The figure shows three views and two pictorial views of one solid part (mm, origin at its lowest corner). Answer the questions. Give positions to 0.01 mm unless a question says otherwise; leave off trailing zeros. Loops run counter-clockwise (first coordinate to the right, second up) from the corner with the lowest first, then second, coordinate; pieces in that order, holes last. Notation, with made-up numbers: (-9.5, 62) - (31.5, 62) arc R23 cw to (31.5, 83) - close; hole circle Ø5 at (76, 81). An arc over 180 degrees is marked (long way). Use a Markdown table: item, result. Add a question column.
Item 1: For a pull along X with two mould halves and no side action, classify the marked faces 1, 2, 3 and 4 as +X half, -X half, draft (parallel to the pull), parting line (faces both ways), or undercut.
Item 2: Consider probe 1 along X at (y, z) = (2, 19); probe 2 along X at (y, z) = (12, 19.5); probe 3 along X at (y, z) = (48, 18). Determine where each line is inside the solid, lowest interval first. Write a range as [from, to].
Item 3: A cutting plane is placed at A-A (z = 19.05). Determine the outline of the cut face in (x, y) (3 decimals), plus the area to 3 significant figures.
Item 4: A cutting plane is placed at B-B (x = 120.65). Determine the outline of the cut face in (y, z) (3 decimals).
Item 5: Each of these flat-tipped pins is pushed along its axis until it touches: P1, Ø17, axis at x = 120.65, z = 19.05, coming from the -Y side; P2, Ø3, axis at x = 78, z = 17, coming from the -Y side. Where does it stop, or does it pass through?
Item 6: A cutting plane is placed at D-D (y = 21.5). Determine the outline of the cut face in (x, z) (3 decimals), plus the area to 3 significant figures.
Item 7: A cutting plane is placed at C-C (x = 59.69). Determine the outline of the cut face in (y, z).
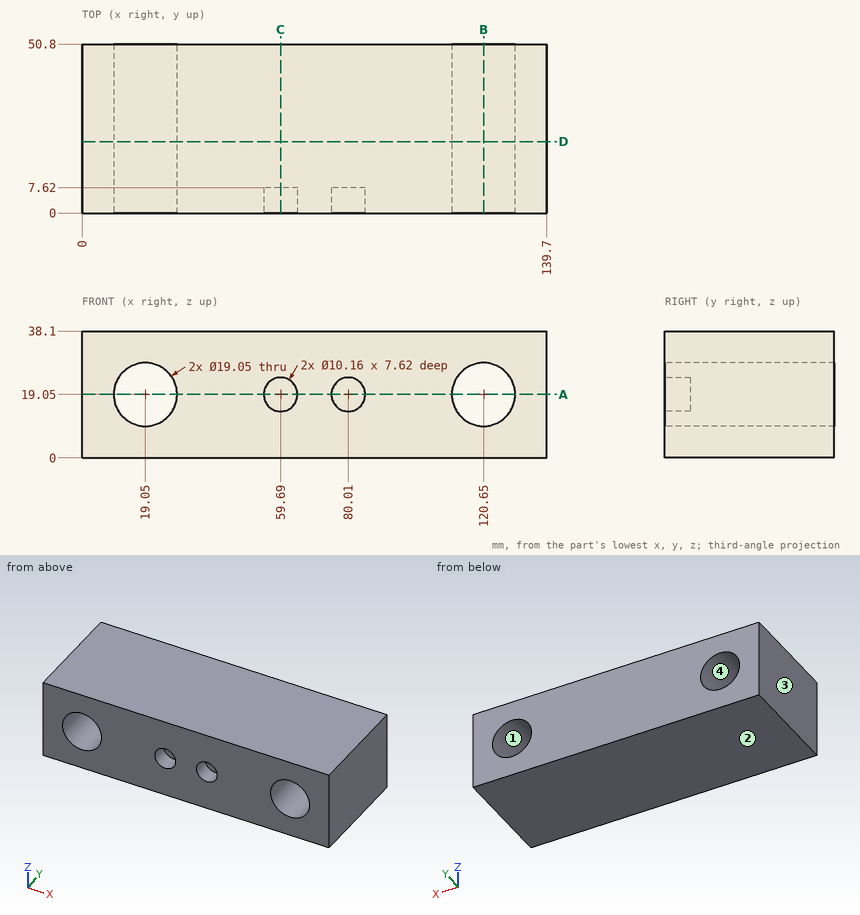
Geometry says:
| question | item | result |
|---|---|---|
| 1 | face 1 | undercut |
| 1 | face 2 | draft |
| 1 | face 3 | -X half |
| 1 | face 4 | undercut |
| 2 | probe 1 | [0, 9.53], [28.57, 54.61], [64.77, 74.93], [85.09, 111.13], [130.17, 139.7] |
| 2 | probe 2 | [0, 9.54], [28.56, 111.14], [130.16, 139.7] |
| 2 | probe 3 | [0, 9.58], [28.52, 111.18], [130.12, 139.7] |
| 3 | outline | (0, 0) - (9.525, 0) - (9.525, 50.8) - (0, 50.8) - close; (28.575, 0) - (54.61, 0) - (54.61, 7.62) - (64.77, 7.62) - (64.77, 0) - (74.93, 0) - (74.93, 7.62) - (85.09, 7.62) - (85.09, 0) - (111.125, 0) - (111.125, 50.8) - (28.575, 50.8) - close; (130.175, 0) - (139.7, 0) - (139.7, 50.8) - (130.175, 50.8) - close |
| 3 | area | 5,010 mm² |
| 4 | outline | (0, 0) - (50.8, 0) - (50.8, 9.525) - (0, 9.525) - close; (0, 28.575) - (50.8, 28.575) - (50.8, 38.1) - (0, 38.1) - close |
| 5 | P1 | through |
| 5 | P2 | y = 7.62 |
| 6 | outline | (0, 0) - (139.7, 0) - (139.7, 38.1) - (0, 38.1) - close; hole circle Ø19.05 at (19.05, 19.05); hole circle Ø19.05 at (120.65, 19.05) |
| 6 | area | 4,750 mm² |
| 7 | outline | (0, 0) - (50.8, 0) - (50.8, 38.1) - (0, 38.1) - (0, 24.13) - (7.62, 24.13) - (7.62, 13.97) - (0, 13.97) - close |
